Geometry check sheet. Reference: the model listing, model coordinates, mm. A direction names the side the tool comes from. Give positions to 0.01 mm unless a question says otherwise; leave off trailing zeros. Order: outer loops, then holes, each group sorted by start corner. A loop starts at its lowest first (then second) coordinate and runs counter-clockwise, first axis right, second up.
from build123d import *

# Parameters (mm, degrees)
ESBO_O1_R                = 25
RESSALTO_EXTRUS_O1_DEPTH = 10
ESBO_O2_W                = 2.5
ESBO_O2_H                = 5.2
ESBO_O2_W_2              = 5.2
ESBO_O2_H_2              = 2.5
CORTE_EXTRUS_O1_DEPTH    = 6
ESBO_O3_R                = 0.5
CORTE_EXTRUS_O2_DEPTH    = 0.2


with BuildPart() as part:
    # Esboço1 → Ressalto-extrusão1 (new body)
    with BuildSketch(Plane(origin=(0, 0, 0), x_dir=(1, 0, 0), z_dir=(0, 1, 0))):
        Circle(ESBO_O1_R)
    extrude(amount=RESSALTO_EXTRUS_O1_DEPTH)

    # Esboço2 → Corte-extrusão1 (cut)
    with BuildSketch(Plane.XZ):
        with Locations((-3.85, 0)):
            Rectangle(ESBO_O2_W, ESBO_O2_H)
        Rectangle(ESBO_O2_W_2, ESBO_O2_H)
        with Locations((0, 3.85)):
            Rectangle(ESBO_O2_W_2, ESBO_O2_H_2)
        with Locations((3.85, 0)):
            Rectangle(ESBO_O2_W, ESBO_O2_H)
        with Locations((0, -3.85)):
            Rectangle(ESBO_O2_W_2, ESBO_O2_H_2)
    extrude(amount=-CORTE_EXTRUS_O1_DEPTH, mode=Mode.SUBTRACT)

    # Esboço3 → Corte-extrusão2 (cut)
    with BuildSketch(Plane(origin=(0, 10, 0), x_dir=(1, 0, 0), z_dir=(0, 1, 0))):
        Circle(ESBO_O3_R)
    extrude(amount=-CORTE_EXTRUS_O2_DEPTH, mode=Mode.SUBTRACT)


solid = part.part
Item 1: Set-up check for faces 4 (the flat face through (0, 0, -6)), 5 (the flat face through (-5.1, 3, 0)): record each of +Z, -Z, +X, -X, +Y, -Y from which the full face is reachable in a straight line by a thin tool's end or side.
Reported:
face 4: +Z, -Z, +X, -X, -Y
face 5: -Y
Item 2: Draft check along Z on faces 1 (the flat face through (2.6, 3, 4)), 2 (the cylindrical face through (23.846, 4.93, -7.509)), 3 (the flat face through (0, 10, 5)). Enter one of: released by +Z, released by -Z, zero draft, split by the parting line, or undercut.
Reported:
face 1: undercut
face 2: split by the parting line
face 3: zero draft
Item 3: Sectioned sample at D-D (x = -9). Enter the section's corners in (y, z), and give its area (3 significant figures).
Reported:
outline: (0, -23.32) - (10, -23.32) - (10, 23.32) - (0, 23.32) - close
area: 466 mm2
Item 4: Gauge pin test, flat ends, axial feed: pin 1 (1.2 mm diameter, centred on x = 3.5, y = 3, fed in from +Z); pin 2 (2 mm diameter, centred on y = 3, z = -3.5, fed in from -X); pin 3 (2.5 mm diameter, centred on x = 4.5, y = 2, fed in from -Z). Record the tip position at first contact, or that the pin passes through.
Reported:
pin 1: stops at z = 24.83
pin 2: stops at x = -24.87
pin 3: stops at z = -24.79
Item 5: Sectioned sample at C-C (x = 15). Enter the section's corners in (y, z), and give its area (3 significant figures).
Reported:
outline: (0, -20) - (10, -20) - (10, 20) - (0, 20) - close
area: 400 mm2
Item 6: Scan lines: L1, parallel to Z at x = 0, y = 9.9; L2, parallel to Z at x = 0, y = 2.5; L3, parallel to X at y = 5.25, z = -11.5. Record each from-to range of solid material in increasing order.
Reported:
L1: z = -25 to -0.5, 0.5 to 25
L2: z = -25 to -5.1, 5.1 to 25
L3: x = -22.2 to 22.2
Item 7: Sectioned sample at A-A (z = 4.5). Enter the section's corners in (x, y), and give its area (3 significant figures).
Reported:
outline: (-24.59, 0) - (-2.6, 0) - (-2.6, 6) - (2.6, 6) - (2.6, 0) - (24.59, 0) - (24.59, 10) - (-24.59, 10) - close
area: 461 mm2
Item 8: Sectioned sample at B-B (y = 6.75). Enter the section's corners in (x, z), and give its area (3 significant figures).
Reported:
outline: circle Ø50 at (0, 0)
area: 1,960 mm2
